CAD build for the part. Positions are in the model's coordinates, mm. A direction names the side the tool comes from. Give positions to 0.01 mm unless a question says otherwise; leave off trailing zeros. Write each loop counter-clockwise with the first axis right and the second up, starting at its lowest first coordinate (ties: lowest second). Pieces come first, ordered by that corner, then holes. Notation, with made-up numbers: (58.25, 78) - (80.25, 78) arc R11 cw to (80.25, 90) - close; hole circle Ø9 at (-27, 75). An arc over 180 degrees is marked (long way). Put each result on its own line as item: value. Start each with the question number.
1. Cut at D-D on x = -13.5. List the corners of the cut face in (y, z), and give its area (3 significant figures).
2. Tool access for faces 4 (the flat face through (50, -70, 8)), 5 (the flat face through (-1, 0, -2)): list every direction of +Z, -Z, +X, -X, +Y, -Y with a clear straight run to the whole face (end or side of a thin tool).
3. Mould opens along X. For faces 1 (the cylindrical face through (-39.077, -161.774, 8.521)), 2 (the flat face through (-1, -84, 7)), 3 (the flat face through (-50, -70, 8)) say: +X half, -X half, draft (parallel to the pull), parting line (faces both ways), or undercut.
4. Cut at C-C on x = -40. List the corners of the cut face in (y, z), and give its area (3 significant figures).
5. Drop flat-ended pins along their axis: pin 1 (8.5 mm diameter, centred on x = -10.5, z = -5.5, fed in from -Y); pin 2 (1 mm diameter, centred on x = -8.5, y = -23.5, fed in from -Z); pin 3 (2.5 mm diameter, centred on x = 40, z = 0, fed in from +Y). Give the stop position or say it passes through.
6. Cut at A-A on z = 0. List the corners of the cut face in (x, y), and give its area (3 significant figures).
7. Wall check: line 1 (X direction, y = 1.45, z = 0); line 2 (Y direction, x = 40, z = 8.05); line 3 (Z direction, x = 45, y = -102). Give the ranges that are in metal, low to high.
8. Cut at B-B on y = -160. List the corners of the cut face in (x, z).
from build123d import *

# Parameters (mm, degrees)
SKETCH1_W           = 100
SKETCH1_H           = 20
BOSS_EXTRUDE1_DEPTH = 3
CUT_EXTRUDE1_REACH  = 53.078
SKETCH2_R           = 2
SKETCH3_W           = 100
SKETCH3_H           = 3
BOSS_EXTRUDE2_DEPTH = 170
CUT_EXTRUDE2_REACH  = 180.326
SKETCH4_R           = 2


with BuildPart() as part:
    # Sketch1 → Boss-Extrude1 (new body)
    with BuildSketch(Plane(origin=(0, 0, 0), x_dir=(1, 0, 0), z_dir=(0, 1, 0))):
        Rectangle(SKETCH1_W, SKETCH1_H)
    extrude(amount=BOSS_EXTRUDE1_DEPTH)

    # Sketch2 → Cut-Extrude1 (cut, up to next)
    with BuildSketch(Plane(origin=(0, 3, 0), x_dir=(1, 0, 0), z_dir=(0, 1, 0)), mode=Mode.PRIVATE) as cut_extrude1_sk1:
        with Locations(Location((40, 0, 0), (0, 0, 270))):
            Circle(SKETCH2_R)
    cut_extrude1_tool1 = extrude(cut_extrude1_sk1.sketch, amount=-CUT_EXTRUDE1_REACH, mode=Mode.PRIVATE) & part.part
    # Sketch2 → Cut-Extrude1 (cut, up to next)
    with BuildSketch(Plane(origin=(0, 3, 0), x_dir=(1, 0, 0), z_dir=(0, 1, 0)), mode=Mode.PRIVATE) as cut_extrude1_sk2:
        with Locations(Location((-40, 0, 0), (0, 0, 270))):
            Circle(SKETCH2_R)
    cut_extrude1_tool2 = extrude(cut_extrude1_sk2.sketch, amount=-CUT_EXTRUDE1_REACH, mode=Mode.PRIVATE) & part.part
    add(cut_extrude1_tool1.solids().sort_by_distance((40, 3, 0))[0], mode=Mode.SUBTRACT)
    add(cut_extrude1_tool2.solids().sort_by_distance((-40, 3, 0))[0], mode=Mode.SUBTRACT)

    # Sketch3 → Boss-Extrude2 (add)
    with BuildSketch(Plane.XZ):
        with Locations((0, 8.5)):
            Rectangle(SKETCH3_W, SKETCH3_H)
    extrude(amount=BOSS_EXTRUDE2_DEPTH)

    # Sketch4 → Cut-Extrude2 (cut, up to next)
    with BuildSketch(Plane.XY.offset(10), mode=Mode.PRIVATE) as cut_extrude2_sk1:
        with Locations((-40, -160)):
            Circle(SKETCH4_R)
    cut_extrude2_tool1 = extrude(cut_extrude2_sk1.sketch, amount=-CUT_EXTRUDE2_REACH, mode=Mode.PRIVATE) & part.part
    # Sketch4 → Cut-Extrude2 (cut, up to next)
    with BuildSketch(Plane.XY.offset(10), mode=Mode.PRIVATE) as cut_extrude2_sk2:
        with Locations((40, -160)):
            Circle(SKETCH4_R)
    cut_extrude2_tool2 = extrude(cut_extrude2_sk2.sketch, amount=-CUT_EXTRUDE2_REACH, mode=Mode.PRIVATE) & part.part
    add(cut_extrude2_tool1.solids().sort_by_distance((-40, -160, 10))[0], mode=Mode.SUBTRACT)
    add(cut_extrude2_tool2.solids().sort_by_distance((40, -160, 10))[0], mode=Mode.SUBTRACT)


solid = part.part
Report:
1. outline: (-170, 7) - (0, 7) - (0, -10) - (3, -10) - (3, 10) - (-170, 10) - close
1. area: 570 mm²
2. face 4: +Z, -Z, +X, +Y, -Y
2. face 5: -Z, +X, -X, -Y
3. face 1: undercut
3. face 2: draft
3. face 3: -X half
4. outline: (-170, 7) - (-162, 7) - (-162, 10) - (-170, 10) - close; (-158, 7) - (0, 7) - (0, 2) - (3, 2) - (3, 10) - (-158, 10) - close; (0, -10) - (3, -10) - (3, -2) - (0, -2) - close
4. area: 546 mm²
5. pin 1: stops at y = 0
5. pin 2: stops at z = 7
5. pin 3: passes through
6. outline: (-50, 0) - (-42, 0) - (-42, 3) - (-50, 3) - close; (-38, 0) - (38, 0) - (38, 3) - (-38, 3) - close; (42, 0) - (50, 0) - (50, 3) - (42, 3) - close
6. area: 276 mm²
7. line 1: x = -50 to -42, -38 to 38, 42 to 50
7. line 2: y = -170 to -162, -158 to 3
7. line 3: z = 7 to 10
8. outline: (-50, 7) - (-42, 7) - (-42, 10) - (-50, 10) - close; (-38, 7) - (38, 7) - (38, 10) - (-38, 10) - close; (42, 7) - (50, 7) - (50, 10) - (42, 10) - close
